from build123d import *

# Parameters (mm, degrees)
BOSS_EXTRU_2_DEPTH       = 42
BOSS_EXTRU_3_DEPTH       = 3
CONG_5_R                 = 1
CONG_6_R                 = 3
CONG_7_R                 = 3
ESQUISSE4_R              = 4.6
ENL_V_MAT_EXTRU_1_DEPTH  = 1.6
ESQUISSE5_R              = 2.5
ENL_V_MAT_EXTRU_2_DEPTH  = 4
ESQUISSE6_R              = 4.6
ENL_V_MAT_EXTRU_3_DEPTH  = 1.6
ESQUISSE7_R              = 2.5
ENL_V_MAT_EXTRU_4_DEPTH  = 4
ENL_V_MAT_EXTRU_8_DEPTH  = 1.2
BOSS_EXTRU_4_DEPTH       = 8
ESQUISSE14_R             = 6.1
ENL_V_MAT_EXTRU_9_DEPTH  = 4
ENL_V_MAT_EXTRU_11_DEPTH = 3


with BuildPart() as part:
    # Esquisse1 → Boss.-Extru.2 (new body)
    with BuildSketch(Plane.XY):
        Polygon((-73, 90.945896367), (-28.961701152, 153.839105087), (28.961701152, 153.839105087), (73, 90.945896367), (73, -3), (-73, -3), align=None)
        Polygon((70, 0), (-70, 0), (-70, 90), (-27.4, 150.839105087), (27.4, 150.839105087), (70, 90), align=None, mode=Mode.SUBTRACT)
    extrude(amount=BOSS_EXTRU_2_DEPTH)

    # Esquisse3 → Boss.-Extru.3 (add)
    with BuildSketch(Plane.XY):
        Polygon((-70, 90), (-27.4, 150.839105087), (27.4, 150.839105087), (70, 90), (70, 0), (-70, 0), align=None)
    extrude(amount=BOSS_EXTRU_3_DEPTH)

    # Congé5
    cong_5_edges = [part.edges().sort_by_distance(p)[0] for p in [
        (70, 0, 22.5),
        (70, 90, 22.5),
        (27.4, 150.839105087, 22.5),
        (-27.4, 150.839105087, 22.5),
        (-70, 90, 22.5),
        (-70, 0, 22.5),
    ]]
    fillet(cong_5_edges, radius=CONG_5_R)

    # Congé6
    cong_6_edges = [part.edges().sort_by_distance(p)[0] for p in [
        (-73, -3, 21),
        (73, -3, 21),
        (73, 90.945896367, 21),
        (28.961701152, 153.839105087, 21),
        (-28.961701152, 153.839105087, 21),
        (-73, 90.945896367, 21),
    ]]
    fillet(cong_6_edges, radius=CONG_6_R)

    # Congé7
    cong_7_edges = [part.edges().sort_by_distance(p)[0] for p in [
        (-51.157456133, 122.140281853, 0),
        (51.157456133, 122.140281853, 0),
        (73, 45, 0),
        (0, -3, 0),
        (-28.78524584, 153.500137587, 0),
        (-72.861150852, 90.902117399, 0),
        (-72.121320344, -2.121320344, 0),
        (72.121320344, -2.121320344, 0),
        (72.861150852, 90.902117399, 0),
        (28.78524584, 153.500137587, 0),
        (0, 153.839105087, 0),
        (-73, 45, 0),
    ]]
    fillet(cong_7_edges, radius=CONG_7_R)

    # Esquisse4 → Enlèv. mat.-Extru.1 (cut)
    with BuildSketch(Plane(origin=(-70, 0, 0), x_dir=(0, 0, -1), z_dir=(1, 0, 0))):
        with Locations((-13, 26)):
            Circle(ESQUISSE4_R)
    extrude(amount=-ENL_V_MAT_EXTRU_1_DEPTH, mode=Mode.SUBTRACT)

    # Esquisse5 → Enlèv. mat.-Extru.2 (cut, through all)
    with BuildSketch(Plane(origin=(-70, 0, 0), x_dir=(0, 0, -1), z_dir=(1, 0, 0))):
        with Locations((-13, 26)):
            Circle(ESQUISSE5_R)
    extrude(amount=-ENL_V_MAT_EXTRU_2_DEPTH, mode=Mode.SUBTRACT)

    # Esquisse6 → Enlèv. mat.-Extru.3 (cut)
    with BuildSketch(Plane.ZY.offset(-70)):
        with Locations((13, 26)):
            Circle(ESQUISSE6_R)
    extrude(amount=-ENL_V_MAT_EXTRU_3_DEPTH, mode=Mode.SUBTRACT)

    # Esquisse7 → Enlèv. mat.-Extru.4 (cut, through all)
    with BuildSketch(Plane.ZY.offset(-70)):
        with Locations((13, 26)):
            Circle(ESQUISSE7_R)
    extrude(amount=-ENL_V_MAT_EXTRU_4_DEPTH, mode=Mode.SUBTRACT)

    # Esquisse12 → Enlèv. mat.-Extru.8 (cut)
    with BuildSketch(Plane(origin=(0, 153.839105087, 0), x_dir=(1, 0, 0), z_dir=(0, 1, 0))):
        with BuildLine():
            ThreePointArc((24.9, -26.291388692), (0.316807272, -7.658549634), (-24.9, -25.424491407))
            ThreePointArc((-24.9, -25.424491407), (0.10338435, -19.918896621), (24.9, -26.291388692))
        make_face()
    extrude(amount=-ENL_V_MAT_EXTRU_8_DEPTH, mode=Mode.SUBTRACT)

    # Esquisse13 → Boss.-Extru.4 (add)
    with BuildSketch(Plane.ZY.offset(-70)):
        Polygon((3, 89.684701211), (3, 88.684701211), (37.6, 88.684701211), (37.6, 43.084701211), (3, 43.084701211), (3, 42.084701211), (38.6, 42.084701211), (38.6, 89.684701211), align=None)
    extrude(amount=BOSS_EXTRU_4_DEPTH)

    # Esquisse14 → Enlèv. mat.-Extru.9 (cut, through all)
    with BuildSketch(Plane.XY.offset(3)):
        with Locations((0, 26)):
            Circle(ESQUISSE14_R)
    extrude(amount=-ENL_V_MAT_EXTRU_9_DEPTH, mode=Mode.SUBTRACT)

    # Esquisse16 → Enlèv. mat.-Extru.11 (cut)
    with BuildSketch(Plane.XZ.offset(3)):
        with BuildLine():
            Line((-25, 3), (25, 3))
            ThreePointArc((25, 3), (0, 28), (-25, 3))
        make_face()
    extrude(amount=-ENL_V_MAT_EXTRU_11_DEPTH, mode=Mode.SUBTRACT)


solid = part.part
Could you check a few things on this model? Use its own coordinates, in mm. A direction names the side the tool comes from. Give positions to 0.01 mm unless a question says otherwise; leave off trailing zeros. Order: outer loops, then holes, each group sorted by start corner. A loop starts at its lowest first (then second) coordinate and runs counter-clockwise, first axis right, second up. Notation, with made-up numbers: (3, 22.25) - (27, 22.25) arc R25 ccw to (27, 56.25) - close; hole circle Ø11 at (31, 40). An arc over 180 degrees is marked (long way). Return JSON: item names as keys, results as strings. Group by question number.
Q1. Suppose I cut it at C-C, the plane x = 0. Please give me the cut outline in (y, z), and give its area (3 significant figures).
Q2. Suppose I cut it at D-D, the plane y = 84.5. Please give me the cut outline in (x, z).
Q3. Which directions (+Z, -Z, +X, -X, +Y, -Y) give clear straight access to the entire face, cutting with the end or side of a thin tool? Please do faces 3 (the face through (70.79, 29.88, 15.47)), 4 (the face through (70, 26, 27)), 5 (the face through (0, 152.639, 15)), 6 (the face through (0.55, -1.521, 27.994)).
Q4. Thinking about a two-plate mould opening in Z: for faces 1 (the face through (73, 46, 22)), 2 (the face through (70, 66, 20)), which applies, pulls with the +Z half, pulls with the -Z half, needs draft (parallel to the pull), parting line crosses it, or undercut?
Q5. Please list where these lines run through material, in increasing order: line 1 along Y through (x, z) = (24, 16); line 2 along X through (y, z) = (77.5, 19); line 3 along Z through (x, y) = (-4, 70). Write a range as [from, to].
Q6. Suppose I cut it at B-B, the plane y = 26. State how many separate pieces and enclosed holes the cut face has, and give its area (3 significant figures).
Q7. Will these pins go through, and if not, where does the flat tip stop? pin 1 Ø11.5 at (x, z) = (-2, 23) entering from -Y; pin 2 Ø1 at (x, z) = (55, 28) entering from +Y; pin 3 Ø6 at (x, z) = (4, 11.5) entering from -Y; pin 4 Ø6.5 at (x, z) = (68, 18) entering from +Y.
Resolved:
{
 "1": {"outline": "(-3, 3) arc R3 ccw to (0, 0) - (19.9, 0) - (19.9, 3) - close; (-3, 28) - (0, 28) - (0, 42) - (-3, 42) - close; (32.1, 0) - (150.84, 0) arc R3 ccw to (153.84, 3) - (153.84, 7.65) - (152.64, 7.65) - (152.64, 19.92) - (153.84, 19.92) - (153.84, 42) - (150.84, 42) - (150.84, 3) - (32.1, 3) - close", "area": "574 mm2"},
 "2": {"outline": "(-73, 3) arc R3 ccw to (-70, 0) - (70, 0) arc R3 ccw to (73, 3) - (73, 42) - (70, 42) - (70, 38.6) - (62, 38.6) - (62, 37.6) - (70, 37.6) - (70, 3) - (-70, 3) - (-70, 42) - (-73, 42) - close"},
 "3": {"face 3": "none", "face 4": "+Z", "face 5": "+Y", "face 6": "-Y"},
 "4": {"face 1": "needs draft", "face 2": "undercut"},
 "5": {"line 1": "y = [-3, 0], [150.84, 153.84]", "line 2": "x = [-73, -70], [70, 73]", "line 3": "z = [0, 3]"},
 "6": {"separate pieces": "4", "enclosed holes": "0", "area": "588 mm2"},
 "7": {"pin 1": "stops at y = -3", "pin 2": "stops at y = 117.37", "pin 3": "stops at y = 150.84", "pin 4": "stops at y = 102.73"}
}
